Source: CAD feature listing. Evaluate the final solid. Frame: model axes, mm. A direction names the side the tool comes from. Give positions to 0.01 mm unless a question says otherwise; leave off trailing zeros. Loops run counter-clockwise (first coordinate to the right, second up) from the corner with the lowest first, then second, coordinate; pieces in that order, holes last.
```python
from build123d import *

# Parameters (mm, degrees)
F1_DEPTH = 6
F3_DEPTH = 6
F4_W     = 25
F4_H     = 12
F5_DEPTH = 6
F6_D     = 13


with BuildPart() as f1:
    # F0 (on Top) → F1 (new body)
    with BuildSketch(Plane.XY):
        with BuildLine():
            Line((-32, -12.5), (32, -12.5))
            Line((32, -12.5), (32, -6.5))
            Line((32, -6.5), (12, -6.5))
            ThreePointArc((12, -6.5), (5.5, 0), (12, 6.5))
            Line((12, 6.5), (32, 6.5))
            Line((32, 6.5), (32, 12.5))
            Line((32, 12.5), (-32, 12.5))
            Line((-32, 12.5), (-32, -12.5))
        make_face()
    extrude(amount=F1_DEPTH)

    # F2 (on face) → F3 (join)
    with BuildSketch(Plane(origin=(-32, 0, 0), x_dir=(0, -1, 0), z_dir=(-1, 0, 0))):
        with BuildLine():
            ThreePointArc((-12.5, -12), (0, -24.5), (12.5, -12))
            Line((12.5, -12), (6.5, -12))
            ThreePointArc((6.5, -12), (0, -18.5), (-6.5, -12))
            Line((-6.5, -12), (-12.5, -12))
        make_face()
        with BuildLine():
            Line((6.5, -12), (12.5, -12))
            ThreePointArc((12.5, -12), (10, -4.5), (3.5, 0))
            Line((3.5, 0), (-3.5, 0))
            ThreePointArc((-3.5, 0), (-10, -4.5), (-12.5, -12))
            Line((-12.5, -12), (-6.5, -12))
            ThreePointArc((-6.5, -12), (0, -5.5), (6.5, -12))
        make_face()
        with BuildLine():
            Line((12.5, -12), (12.5, 0))
            Line((12.5, 0), (3.5, 0))
            ThreePointArc((3.5, 0), (10, -4.5), (12.5, -12))
        make_face()
        with BuildLine():
            Line((-3.5, 0), (-12.5, 0))
            Line((-12.5, 0), (-12.5, -12))
            ThreePointArc((-12.5, -12), (-10, -4.5), (-3.5, 0))
        make_face()
    extrude(amount=-F3_DEPTH)

    # F4 (on face) → F5 (join)
    with BuildSketch(Plane.XZ.offset(12.5)):
        with Locations((-19.5, 12)):
            Rectangle(F4_W, F4_H)
        with BuildLine():
            ThreePointArc((-7, 18), (-19.5, 30.5), (-32, 18))
            Line((-32, 18), (-7, 18))
        make_face()
    extrude(amount=-F5_DEPTH)

    # F6 (through all)
    with Locations(Plane.XZ.offset(12.5)):
        with Locations((-19.5, 18)):
            Hole(F6_D / 2)


solid = f1.part
```
(1) Section C-C, the plane z = 19.5. Return the cut outline in (x, y), then the cut area to 3 significant figures.
A:
outline: (-31.91, -12.5) - (-25.82, -12.5) - (-25.82, -6.5) - (-31.91, -6.5) - close; (-13.18, -12.5) - (-7.09, -12.5) - (-7.09, -6.5) - (-13.18, -6.5) - close
area: 73.0 mm2
(2) First-contact query: pin 1 (6 mm diameter, centred on x = -24.5, y = -6, fed in from +Z); pin 2 (7.5 mm diameter, centred on y = 2.5, z = -17, fed in from +X); pin 3 (8 mm diameter, centred on x = 23, y = -8.5, fed in from -Z); pin 4 (3 mm diameter, centred on y = -3.5, z = -13, fed in from +X). Flat tips, straight axial feed; report the tip coordinate or a pass-through.
A:
pin 1: stops at z = 30.33
pin 2: stops at x = -26
pin 3: stops at z = 0
pin 4: passes through
(3) Reachability of faces 5 (the flat face through (22, 6.5, 3)), 6 (the flat face through (-4, 0, 0)), 7 (the flat face through (-20, -6.5, 10)) from +Z, -Z, +X, -X, +Y, -Y: full face, straight path, thin tool, end or side. Return the list, or none.
A:
face 5: +Z, -Z, +X
face 6: -Z, +X, +Y, -Y
face 7: +Z, +X, -X, +Y
(4) Section B-B, the plane x = -19.5. Return the cut outline in (y, z).
A:
outline: (-12.5, 0) - (12.5, 0) - (12.5, 6) - (-6.5, 6) - (-6.5, 11.5) - (-12.5, 11.5) - close; (-12.5, 24.5) - (-6.5, 24.5) - (-6.5, 30.5) - (-12.5, 30.5) - close
(5) Mould query, pull axis Y, two halves, no side actions, for faces 1 (the flat face through (-32, 0, -4)), 2 (the flat face through (-8, 12.5, 1)), 3 (the cylindrical face through (-29.042, 0.275, -24.497)), 4 (the flat face through (22, -6.5, 3)). Classes: pulls with the +Y half, pulls with the -Y half, needs draft (parallel to the pull), parting line crosses it, or undercut.
A:
face 1: needs draft
face 2: pulls with the +Y half
face 3: parting line crosses it
face 4: undercut
(6) Section A-A, the plane y = 0. Return the cut outline in (x, z), then the cut area to 3 significant figures.
A:
outline: (-32, -24.5) - (-26, -24.5) - (-26, -18.5) - (-32, -18.5) - close; (-32, -5.5) - (-26, -5.5) - (-26, 0) - (5.5, 0) - (5.5, 6) - (-32, 6) - close
area: 294 mm2
(7) Section D-D, the plane y = -9.25. Return the cut outline in (x, z), then the cut area to 3 significant figures.
A:
outline: (-32, -20.41) - (-26, -20.41) - (-26, 0) - (32, 0) - (32, 6) - (-7, 6) - (-7, 18) arc R12.5 ccw to (-32, 18) - close; hole circle Ø13 at (-19.5, 18)
area: 919 mm2
(8) Ray query, line 1 along Z through (x, y) = (-19.5, -9.8); line 2 along Y through (x, z) = (27, 2); line 3 along X through (y, z) = (7.25, -18.5). Return the intervals inside material, ascending.
A:
line 1: z = 0 to 11.5, 24.5 to 30.5
line 2: y = -12.5 to -6.5, 6.5 to 12.5
line 3: x = -32 to -26
